Check sheet for the modelled part. Datum: model origin and axes. Units: mm. A direction names the side the tool comes from. Give positions to 0.01 mm unless a question says otherwise; leave off trailing zeros. Order: outer loops, then holes, each group sorted by start corner. A loop starts at its lowest first (then second) coordinate and runs counter-clockwise, first axis right, second up.
Item 1: Sectioned sample at A-A on z = 6. Record the boundary of the cut face in (x, y).
Item 2: Sectioned sample at B-B on y = -3.3. Record the boundary of the cut face in (x, z) (3 decimals), and give its area (3 significant figures).
Item 3: Sectioned sample at C-C on x = -1.5. Record the boundary of the cut face in (y, z) (3 decimals), and give its area (3 significant figures).
Item 4: Release check for a two-part mould opening along Z. For faces 1 (the flat face through (1, -2, 16.165)), 2 (the flat face through (16.44, -2, 0)), 3 (the flat face through (-7.25, -2, -5)), 4 (the flat face through (0, -2, -1.85)) record: released by +Z, released by -Z, zero draft, split by the parting line, or undercut.
Item 5: Material ranges on line 1 along Z through (x, y) = (-2.5, -3.3) (3 decimals); line 2 along X through (y, z) = (-0.4, -4); line 3 along Z through (x, y) = (-7, -1.55) (3 decimals), recorded low to high.
Item 6: Access from +Z, -Z, +X, -X, +Y, -Y to the whole of each face (thin tool, end or side, straight path). Record for faces 5 (the flat face through (0, -2, 1.85)), 6 (the cylindrical face through (-16.14, -2.12, 15.88)).
from build123d import *

# Parameters (mm, degrees)
F1_DEPTH = 4.3
F2_W     = 14.5
F2_H     = 6.9
F3_DEPTH = 25
F4_R     = 0.5


with BuildPart() as f1:
    # F0 (on Front) → F1 (new body)
    with BuildSketch(Plane.XZ):
        with BuildLine():
            Line((16.44, -16.165), (16.44, 16.165))
            Line((16.44, 16.165), (-15.44, 16.165))
            ThreePointArc((-15.44, 16.165), (-16.147107, 15.872107), (-16.44, 15.165))
            Line((-16.44, 15.165), (-16.44, -15.165))
            ThreePointArc((-16.44, -15.165), (-16.147107, -15.872107), (-15.44, -16.165))
            Line((-15.44, -16.165), (16.44, -16.165))
        make_face()
    extrude(amount=F1_DEPTH)

    # F2 (on face) → F3 (cut)
    with BuildSketch(Plane.XZ.offset(4.3)):
        with Locations((0, 5.3)):
            Rectangle(F2_W, F2_H)
        with Locations((0, -5.3)):
            Rectangle(F2_W, F2_H)
    extrude(amount=-F3_DEPTH, mode=Mode.SUBTRACT)

    # F4
    f4_edges = [f1.edges().sort_by_distance(p)[0] for p in [
        (7.25, -2.15, 8.75),
        (7.25, -2.15, 1.85),
        (-7.25, -2.15, 1.85),
        (-7.25, -2.15, 8.75),
        (-7.25, -2.15, -1.85),
        (7.25, -2.15, -1.85),
        (7.25, -2.15, -8.75),
        (-7.25, -2.15, -8.75),
    ]]
    fillet(f4_edges, radius=F4_R)


solid = f1.part
Report:
1. outline: (-16.44, -4.3) - (-7.25, -4.3) - (-7.25, 0) - (-16.44, 0) - close; (7.25, -4.3) - (16.44, -4.3) - (16.44, 0) - (7.25, 0) - close
2. outline: (-16.44, -15.165) arc R1 ccw to (-15.44, -16.165) - (16.44, -16.165) - (16.44, 16.165) - (-15.44, 16.165) arc R1 ccw to (-16.44, 15.165) - close; hole (-7.25, -8.25) arc R0.5 ccw to (-6.75, -8.75) - (6.75, -8.75) arc R0.5 ccw to (7.25, -8.25) - (7.25, -2.35) arc R0.5 ccw to (6.75, -1.85) - (-6.75, -1.85) arc R0.5 ccw to (-7.25, -2.35) - close; hole (-7.25, 2.35) arc R0.5 ccw to (-6.75, 1.85) - (6.75, 1.85) arc R0.5 ccw to (7.25, 2.35) - (7.25, 8.25) arc R0.5 ccw to (6.75, 8.75) - (-6.75, 8.75) arc R0.5 ccw to (-7.25, 8.25) - close
2. area: 863 mm2
3. outline: (-4.3, -16.165) - (0, -16.165) - (0, -8.75) - (-4.3, -8.75) - close; (-4.3, -1.85) - (0, -1.85) - (0, 1.85) - (-4.3, 1.85) - close; (-4.3, 8.75) - (0, 8.75) - (0, 16.165) - (-4.3, 16.165) - close
3. area: 79.7 mm2
4. face 1: released by +Z
4. face 2: zero draft
4. face 3: undercut
4. face 4: undercut
5. line 1: z = -16.165 to -8.75, -1.85 to 1.85, 8.75 to 16.165
5. line 2: x = -16.44 to -7.25, 7.25 to 16.44
5. line 3: z = -16.165 to -8.683, -1.917 to 1.917, 8.683 to 16.165
6. face 5: +Y, -Y
6. face 6: +Z, -X, +Y, -Y
